Could you check a few things on this model? Use its own coordinates, in mm. A direction names the side the tool comes from. Coordinates: 2 decimals unless noted, no trailing zeros. Order: outer loops, then holes, each group sorted by start corner. A loop starts at its lowest first (then second) coordinate and runs counter-clockwise, first axis right, second up.
```python
from build123d import *

# Parameters (mm, degrees)
F0_R          = 4.8625
F1_DEPTH      = 3.2
F2_R          = 7.9375
F2_R_2        = 4.8625
F3_DEPTH      = 8
F4_R          = 7
F5_R          = 3.175
F6_DEPTH      = 5
F7_R          = 0.995
F8_DEPTH      = 25
F8_DEPTH_BACK = 25


with BuildPart() as f1:
    # F0 (on Top) → F1 (new body)
    with BuildSketch(Plane.XY):
        Circle(F0_R)
    extrude(amount=F1_DEPTH)

    # F2 (on face) → F3 (join)
    with BuildSketch(Plane.XY.offset(3.2)):
        Circle(F2_R)
        Circle(F2_R_2, mode=Mode.SUBTRACT)
        Circle(F2_R_2)
    extrude(amount=F3_DEPTH)

    # F4
    f4_edges = [f1.edges().sort_by_distance(p)[0] for p in [
        (-7.9375, 0, 11.2),
    ]]
    fillet(f4_edges, radius=F4_R)

    # F5 (on Top) → F6 (join)
    with BuildSketch(Plane.XY):
        Circle(F5_R)
    extrude(amount=-F6_DEPTH)

    # F7 (on Top) → F8 (cut, two sides)
    with BuildSketch(Plane.XY) as f8_sk:
        Circle(F7_R)
    extrude(amount=-F8_DEPTH, mode=Mode.SUBTRACT)
    extrude(f8_sk.sketch, amount=F8_DEPTH_BACK, mode=Mode.SUBTRACT)


solid = f1.part
```
Item 1: Suppose I cut it at A-A (z = -3.75). List the corners of the cut face in (x, y) for me (3 decimals), and give its area (3 significant figures).
Item 2: For pin 1 Ø2 at (x, y) = (-2, -1.5) entering from +Z; pin 2 Ø5 at (x, z) = (0.5, -0.5) entering from -Y; pin 3 Ø6 at (x, y) = (3.5, -5) entering from +Z, each with a flat end and sliding along its axis, tell me the tip position at first contact or that it passes through.
Item 3: Which directions (+Z, -Z, +X, -X, +Y, -Y) give clear straight access to the entire face, cutting with the end or side of a thin tool? Please do faces 1 (the face through (1, -3.2, 0)), 2 (the face through (1, 1, -5)).
Item 4: I need wall thicknesses on line 1 (Y direction, x = 0, z = -2.85) (3 decimals); line 2 (Y direction, x = 0, z = 3.75) (1 decimal); line 3 (X direction, y = 2, z = 6.75). Which ranges of each line are inside material? Lowest first, please.
Geometry results:
1. outline: circle Ø6.35 at (0, 0); hole circle Ø1.99 at (0, 0)
1. area: 28.6 mm2
2. pin 1: stops at z = 11.18
2. pin 2: stops at y = -4.86
2. pin 3: stops at z = 10.86
3. face 1: -Z
3. face 2: -Z, +X, -X, +Y, -Y
4. line 1: y = -3.175 to -0.995, 0.995 to 3.175
4. line 2: y = -7.9 to -1, 1 to 7.9
4. line 3: x = -7.18 to 7.18
